from build123d import *

# Parameters (mm, degrees)
ESQUISSE1_W             = 208
ESQUISSE1_H             = 220
BOSS_EXTRU_1_DEPTH      = 3
ESQUISSE2_W             = 10
ESQUISSE2_H             = 3
ENL_V_MAT_EXTRU_1_DEPTH = 3


with BuildPart() as part:
    # Esquisse1 → Boss.-Extru.1 (new body)
    with BuildSketch(Plane.XY):
        Rectangle(ESQUISSE1_W, ESQUISSE1_H)
    extrude(amount=BOSS_EXTRU_1_DEPTH)

    # Esquisse2 → Enlèv. mat.-Extru.1 (cut)
    with BuildSketch(Plane.XY.offset(3)):
        with Locations((-104, 108.5)):
            Rectangle(ESQUISSE2_W, ESQUISSE2_H)
        with Locations((-74, 108.5)):
            Rectangle(ESQUISSE2_W, ESQUISSE2_H)
        with Locations((-44, 108.5)):
            Rectangle(ESQUISSE2_W, ESQUISSE2_H)
        with Locations((-14, 108.5)):
            Rectangle(ESQUISSE2_W, ESQUISSE2_H)
        with Locations((16, 108.5)):
            Rectangle(ESQUISSE2_W, ESQUISSE2_H)
        with Locations((46, 108.5)):
            Rectangle(ESQUISSE2_W, ESQUISSE2_H)
        with Locations((76, 108.5)):
            Rectangle(ESQUISSE2_W, ESQUISSE2_H)
        with Locations((106, 108.5)):
            Rectangle(ESQUISSE2_W, ESQUISSE2_H)
        with Locations((106, -108.5)):
            Rectangle(ESQUISSE2_W, ESQUISSE2_H)
        with Locations((76, -108.5)):
            Rectangle(ESQUISSE2_W, ESQUISSE2_H)
        with Locations((46, -108.5)):
            Rectangle(ESQUISSE2_W, ESQUISSE2_H)
        with Locations((16, -108.5)):
            Rectangle(ESQUISSE2_W, ESQUISSE2_H)
        with Locations((-14, -108.5)):
            Rectangle(ESQUISSE2_W, ESQUISSE2_H)
        with Locations((-44, -108.5)):
            Rectangle(ESQUISSE2_W, ESQUISSE2_H)
        with Locations((-74, -108.5)):
            Rectangle(ESQUISSE2_W, ESQUISSE2_H)
        with Locations((-104, -108.5)):
            Rectangle(ESQUISSE2_W, ESQUISSE2_H)
    extrude(amount=-ENL_V_MAT_EXTRU_1_DEPTH, mode=Mode.SUBTRACT)


solid = part.part
Read the model definition and answer for the solid it produces. Units are mm, in the model's axes. Give positions to 0.01 mm unless a question says otherwise; leave off trailing zeros. Write each loop counter-clockwise with the first axis right and the second up, starting at its lowest first coordinate (ties: lowest second). Pieces come first, ordered by that corner, then holes. Notation, with made-up numbers: (89, -15) - (126, -15) arc R27 ccw to (126, 20) - close; hole circle Ø9 at (19.25, -1). An arc over 180 degrees is marked (long way). Return JSON: item names as keys, results as strings.
Q1. Given P1, Ø1.5, axis at y = -108, z = 2, coming from the +X side; P2, Ø0.9, axis at x = -15, z = 1.5, coming from the -Y side; P3, Ø0.9, axis at y = 108, z = 1.5, coming from the -X side, each flat-ended and moving along its own axis, determine where each tip first touches the part or whether it passes through.
Reply:
{"P1": "x = 101", "P2": "y = -107", "P3": "x = -99"}
Q2. Consider line 1 along Y through (x, z) = (47.5, 2.3). Determine where the line is inside the solid, lowest interval first. Write a range as [from, to].
Reply:
{"line 1": "[-107, 107]"}
Q3. A cutting plane is placed at A-A, the plane x = 78.5. Determine the outline of the cut face in (y, z).
Reply:
{"outline": "(-107, 0) - (107, 0) - (107, 3) - (-107, 3) - close"}
